from build123d import *

# Parameters (mm, degrees)
F0_R     = 10.95
F1_DEPTH = 4
F2_SIZE  = 2


with BuildPart() as f1:
    # F0 (on Top) → F1 (new body, symmetric)
    with BuildSketch(Plane.XY):
        Polygon((-7.130276, 39), (-14.260552, 26.65), (-12.471705, 23.551626), (-15.848265, 9.15), (-26.632159, -0.975), (-30.209853, -0.975), (-37.340129, -13.325), (-30.209853, -25.675), (-15.949301, -25.675), (-14.160454, -22.576626), (0, -18.3), (14.160454, -22.576626), (15.949301, -25.675), (30.209853, -25.675), (37.340129, -13.325), (30.209853, -0.975), (26.632159, -0.975), (15.848265, 9.15), (12.471705, 23.551626), (14.260552, 26.65), (7.130276, 39), align=None)
        Polygon((-18.258702, -4.975), (-13.437828, -13.325), (-18.258702, -21.675), (-27.900452, -21.675), (-32.721327, -13.325), (-27.900452, -4.975), align=None, mode=Mode.SUBTRACT)
        Polygon((13.437828, -13.325), (18.258702, -4.975), (27.900452, -4.975), (32.721327, -13.325), (27.900452, -21.675), (18.258702, -21.675), align=None, mode=Mode.SUBTRACT)
        Circle(F0_R, mode=Mode.SUBTRACT)
        Polygon((9.641749, 26.65), (4.820875, 18.3), (-4.820875, 18.3), (-9.641749, 26.65), (-4.820875, 35), (4.820875, 35), align=None, mode=Mode.SUBTRACT)
    extrude(amount=F1_DEPTH, both=True)

    # F2
    f2_edges = [f1.edges().sort_by_distance(p)[0] for p in [
        (10.695414, 32.825, 4),
        (0, 39, 4),
        (-10.695414, 32.825, 4),
        (-13.366128, 25.100813, 4),
        (13.366128, 25.100813, 4),
        (14.159985, 16.350813, 4),
        (21.240212, 4.0875, 4),
        (28.421006, -0.975, 4),
        (33.774991, -7.15, 4),
        (33.774991, -19.5, 4),
        (23.079577, -25.675, 4),
        (7.080227, -20.438313, 4),
        (-7.080227, -20.438313, 4),
        (-15.054878, -24.125813, 4),
        (15.054878, -24.125813, 4),
        (-23.079577, -25.675, 4),
        (-33.774991, -19.5, 4),
        (-33.774991, -7.15, 4),
        (-21.240212, 4.0875, 4),
        (-14.159985, 16.350813, 4),
        (-28.421006, -0.975, 4),
        (-21.240212, 4.0875, -4),
        (-14.159985, 16.350813, -4),
        (-13.366128, 25.100813, -4),
        (-10.695414, 32.825, -4),
        (0, 39, -4),
        (10.695414, 32.825, -4),
        (13.366128, 25.100813, -4),
        (14.159985, 16.350813, -4),
        (21.240212, 4.0875, -4),
        (28.421006, -0.975, -4),
        (33.774991, -7.15, -4),
        (33.774991, -19.5, -4),
        (23.079577, -25.675, -4),
        (15.054878, -24.125813, -4),
        (7.080227, -20.438313, -4),
        (-7.080227, -20.438313, -4),
        (-15.054878, -24.125813, -4),
        (-23.079577, -25.675, -4),
        (-33.774991, -19.5, -4),
        (-33.774991, -7.15, -4),
        (-28.421006, -0.975, -4),
    ]]
    chamfer(f2_edges, length=F2_SIZE)


solid = f1.part
Work out the finished part from the listing and answer in its coordinate system (mm). A direction names the side the tool comes from. Round coordinates to 2 decimals unless told otherwise and drop trailing zeros. Loops run counter-clockwise (first coordinate to the right, second up) from the corner with the lowest first, then second, coordinate; pieces in that order, holes last. Notation, with made-up numbers: (-2.75, -29) - (5.25, -29) arc R28 ccw to (5.25, -7) - close; hole circle Ø7 at (-8.5, -18). An arc over 180 degrees is marked (long way). One line per item, written item: value.
Q1. Each of these flat-tipped pins is pushed along its axis until it touches: pin 1 Ø1 at (y, z) = (-12.5, 1.5) entering from +X; pin 2 Ø1.1 at (x, z) = (-28.5, -0.5) entering from +Y (3 decimals); pin 3 Ø4 at (x, z) = (-10.5, 0) entering from +Y. Where does it stop, or does it pass through?
Check values:
pin 1: x = 37.15
pin 2: y = -0.975
pin 3: y = 36.63
Q2. Find section A-A on y = -4. Give the vertices of the cut face in (x, z).
Check values:
outline: (-31.96, -2) - (-29.65, -4) - (-10.19, -4) - (-10.19, 4) - (-29.65, 4) - (-31.96, 2) - close; (10.19, -4) - (29.65, -4) - (31.96, -2) - (31.96, 2) - (29.65, 4) - (10.19, 4) - close
Q3. The mould has two halves that part along X. Classify faces 1 (the flat face through (15.72, -23.249, 3.014)), 2 (the flat face through (12.275, 25.238, -3.014)), 3 (the flat face through (22.98, -24.661, -3.014)): +X half, -X half, draft (parallel to the pull), parting line (faces both ways), or undercut.
Check values:
face 1: undercut
face 2: +X half
face 3: draft
Q4. For faces 4 (the flat face through (-27.995, -1.989, -3.014)), 5 (the flat face through (-12.33, 25.277, 2.986)), 6 (the flat face through (15.882, -17.558, 0.056)), determine the directions among +Z, -Z, +X, -X, +Y, -Y from which every point of the face is accessible in a straight line to the end or side of a thin tool.
Check values:
face 4: -Z, -X, +Y
face 5: +Z, -X
face 6: +Z, -Z
Q5. Find section D-D on z = -1. State how many separate pieces and enclosed holes the cut face has, and give its area (3 significant figures).
Check values:
separate pieces: 1
enclosed holes: 4
area: 1,600 mm2
Q6. Find section C-C on y = 15. Give the vertices of the cut face in (x, z), and give its area (3 significant figures).
Check values:
outline: (-14.48, -2) - (-12.42, -4) - (12.42, -4) - (14.48, -2) - (14.48, 2) - (12.42, 4) - (-12.42, 4) - (-14.48, 2) - close
area: 223 mm2
Q7. Straight lines are drawn through the part: probe 1 along Y at (x, z) = (0, 0.25); probe 2 along Y at (x, z) = (5.5, -3); probe 3 along X at (y, z) = (-13, 0.5). For each, find the intervals that lie inside material, in ascending order.
Check values:
probe 1: -18.3 to -10.95, 10.95 to 18.3, 35 to 39
probe 2: -18.92 to -9.47, 9.47 to 19.48, 33.82 to 38
probe 3: -37.15 to -32.53, -13.63 to 13.63, 32.53 to 37.15
Q8. Find section B-B on x = -1.5. Give the vertices of the cut face in (y, z).
Check values:
outline: (-18.75, -2) - (-16.66, -4) - (-10.85, -4) - (-10.85, 4) - (-16.66, 4) - (-18.75, 2) - close; (10.85, -4) - (18.3, -4) - (18.3, 4) - (10.85, 4) - close; (35, -4) - (37, -4) - (39, -2) - (39, 2) - (37, 4) - (35, 4) - close
